Autodesk Inventor part; units mm, degrees
ref_plane "YZ Plane" through (0, 0, 0) normal (1, 0, 0) x (0, 1, 0)
ref_plane "XZ Plane" through (0, 0, 0) normal (0, 1, 0) x (-1, 0, 0)
ref_plane "XY Plane" through (0, 0, 0) normal (0, 0, 1) x (1, 0, 0)
sketch "Sketch1" plane through (0, 0, 0) normal (0, 1, 0) x (-1, 0, 0)
  circle A0 centre (0, 0) radius 265
  circle A1 centre (0, 0) radius 335
  line L0 (335, 0) -> (265, 0)
  line L1 (-265, 0) -> (-335, 0)
  line L2 (0, 265) -> (0, 335)
  point P0 (300, 0)
  point P1 (-300, 0)
  point P2 (0, 300)
  dimension "d1" = 670
  dimension "d4" = 530
extrude "Extrusion1" add sketch "Sketch1" along normal blind 6 contours L0 A1 L1 A0 | A0 L2 A1 L0 | A0 L1 A1 L2
sketch "Sketch2" plane through (0, 0, 0) normal (0, -1, 0) x (1, 0, 0)
  circle A0 centre (0, 0) radius 335
  circle A1 centre (0, 0) radius 265
  circle A2 centre (48.4947, 306.1834) radius 11.5
  circle A3 centre (0, 0) radius 265
  line L0 (48.4947, 306.1834) -> (0, 0)
  point P0 (0, 265)
  point P1 (265, 0)
  dimension "d5" = 310
  dimension "d7" = 23
extrude "Cut1" cut sketch "Sketch2" against normal blind 12 contours A2
pattern_circular "Circular Pattern1" count 20 over 360 about axis through (0, 0, 0) along (0, 1, 0) of "Cut1"
equation "\"d9\" = Thickness"
equation "\"BendRadius\" = Thickness"
equation "\"BendReliefWidth\" = Thickness"
equation "\"BendReliefDepth\" = 0.5 * Thickness"
equation "\"CornerReliefSize\" = 4 * Thickness"
equation "\"MinimumRemnant\" = 2 * Thickness"
equation "\"TransitionRadius\" = BendRadius"
equation "\"JacobiRadiusSize\" = BendRadius"
equation "\"GapSize\" = Thickness"
equation "\"d8\" = Thickness"
properties part number "ANP 1403 accses hatch flange" material "Steel"
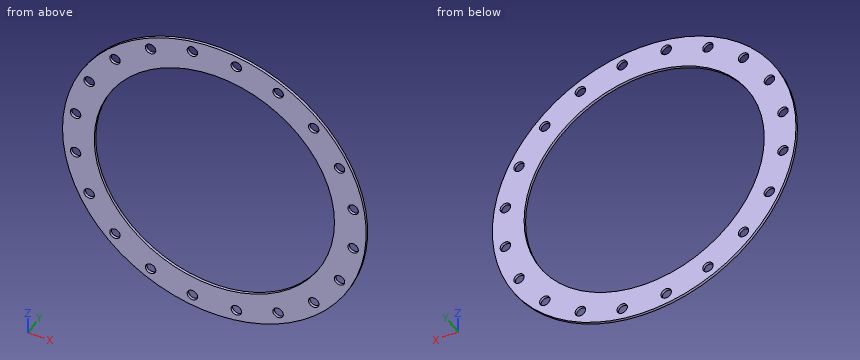
The listing builds one solid part. Answer for the finished solid, in the listing's coordinates (mm). Round coordinates to 2 decimals unless told otherwise and drop trailing zeros. Loops run counter-clockwise (first coordinate to the right, second up) from the corner with the lowest first, then second, coordinate; pieces in that order, holes last.
1) A cutting plane is placed at A-A on x = 0. Determine the outline of the cut face in (y, z).
Outcome:
outline: (0, -335) - (6, -335) - (6, -265) - (0, -265) - close; (0, 265) - (6, 265) - (6, 335) - (0, 335) - close
2) A cutting plane is placed at C-C on y = 3.05. Give the number of separate pieces and of enclosed holes in the cut face, plus the area to 3 significant figures.
Outcome:
separate pieces: 1
enclosed holes: 21
area: 124,000 mm2
3) Given P1, Ø2, axis at x = -208.5, y = 4.5, coming from the +Z side; P2, Ø3, axis at x = 219.5, y = 3, coming from the -Z side; P3, Ø1, axis at x = 191, y = 2, coming from the -Z side, each flat-ended and moving along its own axis, determine where each tip first touches the part or whether it passes through.
Outcome:
P1: stops at z = 263
P2: stops at z = -254.36
P3: stops at z = -275.56
4) Consider line 1 (X direction, y = 1.8, z = -58); line 2 (X direction, y = 5.55, z = 42); line 3 (Z direction, x = 143.5, y = 4.65). Determine where each line is inside the solid, lowest interval first.
Outcome:
line 1: x = -329.94 to -312.66, -299.71 to -258.57, 258.57 to 299.71, 312.66 to 329.94
line 2: x = -332.36 to -315.67, -296.69 to -261.65, 261.65 to 296.69, 315.67 to 332.36
line 3: z = -302.71 to -287.38, -265.05 to -222.78, 222.78 to 265.05, 287.38 to 302.71
5) A cutting plane is placed at B-B on z = 0. Determine the outline of the cut face in (x, y), plus the area to 3 significant figures.
Outcome:
outline: (-335, 0) - (-265, 0) - (-265, 6) - (-335, 6) - close; (265, 0) - (335, 0) - (335, 6) - (265, 6) - close
area: 840 mm2
